from build123d import *

# Parameters (mm, degrees)
SKETCH1_W           = 50.8
SKETCH1_H           = 50.8
BOSS_EXTRUDE1_DEPTH = 863.6
SHELL1_T            = -3.175


with BuildPart() as part:
    # Sketch1 → Boss-Extrude1 (new body)
    with BuildSketch(Plane.XY):
        Rectangle(SKETCH1_W, SKETCH1_H)
    extrude(amount=BOSS_EXTRUDE1_DEPTH)

    # Shell1
    shell1_openings = [part.faces().sort_by_distance(p)[0] for p in [
        (0, 0, 863.6),
        (0, 0, 0),
    ]]
    offset(amount=SHELL1_T, openings=shell1_openings, kind=Kind.INTERSECTION)


solid = part.part
Input: part model. Units: mm. Frame: model coordinates. A direction names the side the tool comes from. Coordinates: 2 decimals unless noted, no trailing zeros. Loops run counter-clockwise (first coordinate to the right, second up) from the corner with the lowest first, then second, coordinate; pieces in that order, holes last.
(1) Pull-direction query (X, two-part tool) for faces 1 (the face through (0, -25.4, 426)), 2 (the face through (22.225, 0, 426)), 3 (the face through (-22.225, 0, 426)), 4 (the face through (-25.4, 0, 426)); classes: released by +X, released by -X, zero draft, split by the parting line, or undercut.
(2) Section C-C on z = 593.5. Return the cut outline in (x, y) (3 decimals), then the cut area to 3 significant figures.
(3) Material intervals for probe 1 along Y at (x, z) = (11.5, 279) (3 decimals), sorted ascending.
(4) Section A-A on y = 7. Return the cut outline in (x, z) (3 decimals).
(5) First-contact query: pin 1 Ø1 at (x, y) = (8, 20) entering from +Z. Flat tip, straight axial feed; report the tip coordinate or a pass-through.
(6) Set-up query: faces 5 (the face through (-23, 0, 0)), 6 (the face through (0, 22.225, 426)). Return all of +Z, -Z, +X, -X, +Y, -Y with unobstructed straight access to the full face (end or side cutting, diameter ignored); none if empty.
Data:
1. face 1: zero draft
1. face 2: undercut
1. face 3: undercut
1. face 4: released by -X
2. outline: (-25.4, -25.4) - (25.4, -25.4) - (25.4, 25.4) - (-25.4, 25.4) - close; hole (-22.225, -22.225) - (22.225, -22.225) - (22.225, 22.225) - (-22.225, 22.225) - close
2. area: 605 mm2
3. probe 1: y = -25.4 to -22.225, 22.225 to 25.4
4. outline: (-25.4, 0) - (-22.225, 0) - (-22.225, 863.6) - (-25.4, 863.6) - close; (22.225, 0) - (25.4, 0) - (25.4, 863.6) - (22.225, 863.6) - close
5. pin 1: passes through
6. face 5: -Z, +X, -X, +Y, -Y
6. face 6: +Z, -Z
